from build123d import *

# Parameters (mm, degrees)
SKETCH1_R           = 3.05
BOSS_EXTRUDE1_DEPTH = 5
FILLET1_R           = 3


with BuildPart() as part:
    # Sketch1 → Boss-Extrude1 (new body)
    with BuildSketch(Plane.XY):
        Polygon((0, 0), (0, 250), (57.43, 250), (278, 27.43), (278, 0), align=None)
        with Locations((15, 210)):
            Circle(SKETCH1_R, mode=Mode.SUBTRACT)
        with Locations((15, 40)):
            Circle(SKETCH1_R, mode=Mode.SUBTRACT)
        with Locations((80, 205.915753479)):
            Circle(SKETCH1_R, mode=Mode.SUBTRACT)
        with Locations((228, 56.573775875)):
            Circle(SKETCH1_R, mode=Mode.SUBTRACT)
    extrude(amount=BOSS_EXTRUDE1_DEPTH)

    # Fillet1
    fillet1_edges = [part.edges().sort_by_distance(p)[0] for p in [
        (0, 0, 2.5),
        (0, 250, 2.5),
        (57.43, 250, 2.5),
        (278, 27.43, 2.5),
        (278, 0, 2.5),
    ]]
    fillet(fillet1_edges, radius=FILLET1_R)


solid = part.part
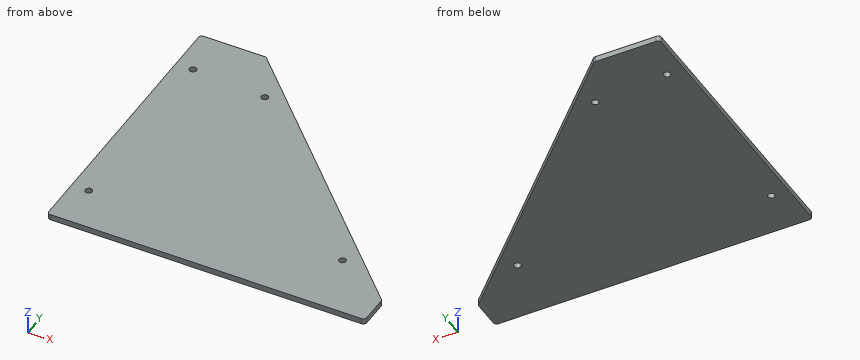
Source: CAD feature listing. Evaluate the final solid. Frame: model axes, mm. Round coordinates to 2 decimals unless told otherwise and drop trailing zeros. Loops run counter-clockwise (first coordinate to the right, second up) from the corner with the lowest first, then second, coordinate; pieces in that order, holes last.
Q1. Ray query, line 1 (Y direction, x = 15, z = 1.55); line 2 (Y direction, x = 16.5, z = 3.9); line 3 (X direction, y = 210, z = 2.55). Return the intervals inside material, ascending.
Q2. First-contact query: P1, Ø10, axis at x = 80, y = 205.92, coming from the +Z side; P2, Ø5.5, axis at x = 228, y = 56.57, coming from the +Z side; P3, Ø3, axis at y = 203, z = 1.5, coming from the +X side. Flat tips, straight axial feed; report the tip coordinate or a pass-through.
Q3. Section B-B, the plane y = 40. Return loops of the section in (x, z).
Q4. Section D-D, the plane y = 133.5. Return loops of the section in (x, z), plus the area to 3 significant figures.
Q5. Section A-A, the plane x = 80. Return loops of the section in (y, z).
Q6. Section C-C, the plane z = 1.25. Return loops of the section in (x, y).
Solutions:
1. line 1: y = 0 to 36.95, 43.05 to 206.95, 213.05 to 250
1. line 2: y = 0 to 37.34, 42.66 to 207.34, 212.66 to 250
1. line 3: x = 0 to 11.95, 18.05 to 97.07
2. P1: stops at z = 5
2. P2: passes through
2. P3: stops at x = 105.49
3. outline: (0, 0) - (11.95, 0) - (11.95, 5) - (0, 5) - close; (18.05, 0) - (265.54, 0) - (265.54, 5) - (18.05, 5) - close
4. outline: (0, 0) - (172.88, 0) - (172.88, 5) - (0, 5) - close
4. area: 864 mm2
5. outline: (0, 0) - (202.87, 0) - (202.87, 5) - (0, 5) - close; (208.97, 0) - (227.23, 0) - (227.23, 5) - (208.97, 5) - close
6. outline: (0, 3) arc R3 ccw to (3, 0) - (275, 0) arc R3 ccw to (278, 3) - (278, 26.2) arc R3 ccw to (277.13, 28.31) - (58.31, 249.11) arc R3 ccw to (56.18, 250) - (3, 250) arc R3 ccw to (0, 247) - close; hole circle Ø6.1 at (15, 40); hole circle Ø6.1 at (15, 210); hole circle Ø6.1 at (80, 205.92); hole circle Ø6.1 at (228, 56.57)
